Read the model definition and answer for the solid it produces. Units are mm, in the model's axes. Face numbers are marked on the shaded views. A direction names the side the tool comes from. Coordinates: 2 decimals unless noted, no trailing zeros. Write each loop counter-clockwise with the first axis right and the second up, starting at its lowest first coordinate (ties: lowest second). Pieces come first, ordered by that corner, then holes. Notation, with made-up numbers: (-33, 33) - (-12, 33) arc R17 cw to (-12, 65) - close; hole circle Ø8 at (45.5, 42). An arc over 180 degrees is marked (long way). Return JSON: item names as keys, results as strings.
```python
from build123d import *

# Parameters (mm, degrees)
BOSS_EXTRUDE1_DEPTH = 36
CUT_EXTRUDE1_DEPTH  = 36
CUT_EXTRUDE2_DEPTH  = 36
SKETCH5_R           = 5.25
CUT_EXTRUDE3_DEPTH  = 107.663020771
CUT_EXTRUDE4_START  = -2
SKETCH6_W           = 68
SKETCH6_H           = 20
SKETCH6_R           = 5.25
CUT_EXTRUDE4_DEPTH  = 2
CUT_EXTRUDE5_START  = -41
CUT_EXTRUDE5_DEPTH  = 41
SKETCH9_R           = 3
CUT_EXTRUDE15_DEPTH = 6
FILLET1_R           = 6
FILLET2_R           = 6
SKETCH11_W          = 20
SKETCH11_H          = 20
CUT_EXTRUDE19_DEPTH = 7
SKETCH13_W          = 20
SKETCH13_H          = 20
CUT_EXTRUDE20_DEPTH = 7


# Read off the part's stored shape, not the designer's step: Cut-Extrude5
with BuildPart() as part:
    # Sketch1 → Boss-Extrude1 (new body)
    with BuildSketch(Plane.XY):
        with BuildLine():
            Line((84, 0), (-84, 0))
            Line((-84, 0), (-80, 14))
            Line((-80, 14), (-43, 14))
            Line((-43, 14), (-43, 55))
            Line((-43, 55), (-22, 55))
            Line((-22, 55), (-22, 43))
            Line((-22, 43), (-19, 43))
            Line((-19, 43), (-19, 40))
            ThreePointArc((-19, 40), (0, 21), (19, 40))
            Line((19, 40), (19, 43))
            Line((19, 43), (22, 43))
            Line((22, 43), (22, 55))
            Line((22, 55), (43, 55))
            Line((43, 55), (43, 14))
            Line((43, 14), (80, 14))
            Line((80, 14), (84, 0))
        make_face()
    extrude(amount=BOSS_EXTRUDE1_DEPTH)

    # Sketch2 → Cut-Extrude1 (cut)
    with BuildSketch(Plane(origin=(0, 14, 0), x_dir=(1, 0, 0), z_dir=(0, 1, 0))):
        with BuildLine():
            Line((60, -13), (68, -13))
            ThreePointArc((68, -13), (73, -18), (68, -23))
            Line((68, -23), (60, -23))
            ThreePointArc((60, -23), (55, -18), (60, -13))
        make_face()
    extrude(amount=-CUT_EXTRUDE1_DEPTH, mode=Mode.SUBTRACT)

    # Sketch4 → Cut-Extrude2 (cut)
    with BuildSketch(Plane(origin=(0, 14, 0), x_dir=(1, 0, 0), z_dir=(0, 1, 0))):
        with BuildLine():
            Line((-60, -23), (-68, -23))
            ThreePointArc((-68, -23), (-73, -18), (-68, -13))
            Line((-68, -13), (-60, -13))
            ThreePointArc((-60, -13), (-55, -18), (-60, -23))
        make_face()
    extrude(amount=-CUT_EXTRUDE2_DEPTH, mode=Mode.SUBTRACT)

    # Sketch5 → Cut-Extrude3 (cut, through all)
    with BuildSketch(Plane(origin=(0, 55, 0), x_dir=(1, 0, 0), z_dir=(0, 1, 0))):
        with Locations(Location((-31, -18, 0), (0, 0, 270))):
            Circle(SKETCH5_R)
        with Locations(Location((31, -18, 0), (0, 0, 90))):
            Circle(SKETCH5_R)
    extrude(amount=-CUT_EXTRUDE3_DEPTH, mode=Mode.SUBTRACT)

    # Sketch6 → Cut-Extrude4 (cut)
    # profile 1 of 2: a face of its own
    with BuildSketch(Plane.XZ.offset(CUT_EXTRUDE4_START)):
        with Locations((-42, 18)):
            Rectangle(SKETCH6_W, SKETCH6_H)
        with Locations(Location((-31, 18, 0), (0, 0, 90))):
            Circle(SKETCH6_R, mode=Mode.SUBTRACT)
        with BuildLine():
            ThreePointArc((-68, 13), (-73, 18), (-68, 23))
            Line((-68, 23), (-60, 23))
            ThreePointArc((-60, 23), (-55, 18), (-60, 13))
            Line((-60, 13), (-68, 13))
        make_face(mode=Mode.SUBTRACT)
    # profile 2 of 2: a face of its own
    with BuildSketch(Plane.XZ.offset(CUT_EXTRUDE4_START)):
        with Locations((42, 18)):
            Rectangle(SKETCH6_W, SKETCH6_H)
        with Locations(Location((31, 18, 0), (0, 0, 270))):
            Circle(SKETCH6_R, mode=Mode.SUBTRACT)
        with BuildLine():
            ThreePointArc((68, 23), (73, 18), (68, 13))
            Line((68, 13), (60, 13))
            ThreePointArc((60, 13), (55, 18), (60, 23))
            Line((60, 23), (68, 23))
        make_face(mode=Mode.SUBTRACT)
    extrude(amount=CUT_EXTRUDE4_DEPTH, mode=Mode.SUBTRACT)

    # Cut-Extrude5 outline → Cut-Extrude5 (cut)
    with BuildSketch(Plane(origin=(0, 55, 0), x_dir=(1, 0, 0), z_dir=(0, 1, 0)).offset(CUT_EXTRUDE5_START)):
        with BuildLine():
            ThreePointArc((43, -18), (42.001212365, -27.214019744), (39.05124838, -36))
            Line((39.05124838, -36), (43, -36))
            Line((43, -36), (43, -18))
        make_face()
        with BuildLine():
            ThreePointArc((39.05124838, 0), (42.001212365, -8.785980256), (43, -18))
            Line((43, -18), (43, 0))
            Line((43, 0), (39.05124838, 0))
        make_face()
        with BuildLine():
            Line((-43, -36), (-39.05124838, -36))
            ThreePointArc((-39.05124838, -36), (-42.001212365, -27.214019744), (-43, -18))
            Line((-43, -18), (-43, -36))
        make_face()
        with BuildLine():
            Line((-43, 0), (-43, -18))
            ThreePointArc((-43, -18), (-42.001212365, -8.785980256), (-39.05124838, 0))
            Line((-39.05124838, 0), (-43, 0))
        make_face()
    extrude(amount=CUT_EXTRUDE5_DEPTH, mode=Mode.SUBTRACT)

    # Sketch9 → Cut-Extrude15 (cut, symmetric)
    with BuildSketch(Plane(origin=(0, 21, 0), x_dir=(1, 0, 0), z_dir=(0, 1, 0))):
        with Locations(Location((0, -18, 0), (0, 0, 270))):
            Circle(SKETCH9_R)
    extrude(amount=CUT_EXTRUDE15_DEPTH, both=True, mode=Mode.SUBTRACT)

    # Fillet1
    fillet1_edges = [part.edges().sort_by_distance(p)[0] for p in [
        (42.001212365, 14, 27.214019744),
    ]]
    fillet(fillet1_edges, radius=FILLET1_R)

    # Fillet2
    fillet2_edges = [part.edges().sort_by_distance(p)[0] for p in [
        (-42.001212365, 14, 27.214019744),
    ]]
    fillet(fillet2_edges, radius=FILLET2_R)

    # Sketch11 → Cut-Extrude19 (cut)
    with BuildSketch(Plane.XZ.offset(-2)):
        with Locations((-31, 18)):
            Rectangle(SKETCH11_W, SKETCH11_H)
    extrude(amount=-CUT_EXTRUDE19_DEPTH, mode=Mode.SUBTRACT)

    # Sketch13 → Cut-Extrude20 (cut)
    with BuildSketch(Plane.XZ.offset(-2)):
        with Locations((31, 18)):
            Rectangle(SKETCH13_W, SKETCH13_H)
    extrude(amount=-CUT_EXTRUDE20_DEPTH, mode=Mode.SUBTRACT)


solid = part.part
```
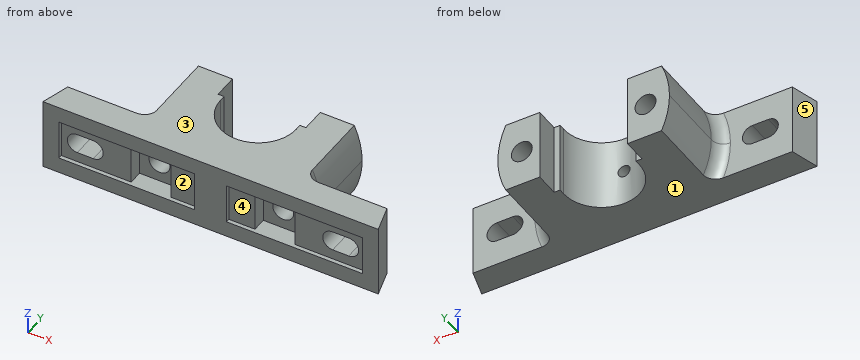
(1) A cutting plane is placed at A-A (x = 31). Determine the outline of the cut face in (y, z), and give its area (3 significant figures).
Answer:
{"outline": "(0, 0) - (55, 0) - (55, 12.75) - (9, 12.75) - (9, 8) - (0, 8) - close; (0, 28) - (9, 28) - (9, 23.25) - (55, 23.25) - (55, 36) - (0, 36) - close", "area": "1,320 mm²"}
(2) Determine the mould class of the marked faces 3, 4 and 5 for opening direction Z: +Z half, -Z half, draft (parallel to the pull), parting line (faces both ways), or undercut.
Answer:
{"face 3": "+Z half", "face 4": "undercut", "face 5": "draft"}
(3) A cutting plane is placed at C-C (x = 0). Determine the outline of the cut face in (y, z).
Answer:
{"outline": "(0, 0) - (21, 0) - (21, 15) - (15, 15) - (15, 21) - (21, 21) - (21, 36) - (0, 36) - close"}
(4) Which of the six approach directions +Z, -Z, +X, -X, +Y, -Y give full straight-line access (tool end or side, diameter ignored) to the marked faces 1 and 2?
Answer:
{"face 1": "-Z, +X, -X, +Y, -Y", "face 2": "-Y"}
(5) Straight lines are drawn through the part: line 1 (X direction, y = 30, z = 22); line 2 (X direction, y = 41, z = 16.5); line 3 (Z direction, x = 0, y = 20.25). For each, find the intervals that lie inside material, in ascending order. Write a range as from..to.
Answer:
{"line 1": "-42.81..-34.4, -27.6..-16.16, 16.16..27.6, 34.4..42.81", "line 2": "-42.97..-36.03, -25.97..-19, 19..25.97, 36.03..42.97", "line 3": "0..15, 21..36"}
(6) Flat-ended cylindrical pins translate along their axes: P1, Ø4, axis at y = 12, z = 21, coming from the -X side; P2, Ø3, axis at y = 39.5, z = 10.5, coming from the +X side; P3, Ø8, axis at x = -59.5, z = 12.5, coming from the +Y side. Find the tip coordinate at first contact, or state that the pin passes through.
Answer:
{"P1": "x = -81.14", "P2": "x = 42.58", "P3": "y = 14"}
(7) A cutting plane is placed at D-D (y = 18.5). Determine the outline of the cut face in (x, z).
Answer:
{"outline": "(-39.26, 0) - (39.26, 0) arc R43.19 ccw to (39.26, 36) - (-39.26, 36) arc R43.19 ccw to start; hole circle Ø10.5 at (-31, 18); hole circle Ø6 at (0, 18); hole circle Ø10.5 at (31, 18)"}
(8) A cutting plane is placed at B-B (y = 34.5). Determine the outline of the cut face in (x, z).
Answer:
{"outline": "(-39.05, 0) - (-18.19, 0) - (-18.19, 36) - (-39.05, 36) arc R43 ccw to start; (18.19, 0) - (39.05, 0) arc R43 ccw to (39.05, 36) - (18.19, 36) - close; hole circle Ø10.5 at (-31, 18); hole circle Ø10.5 at (31, 18)"}
